For this review, take the finished solid that the model builds, in its own axes (mm). Coordinates: 2 decimals unless noted, no trailing zeros. Order: outer loops, then holes, each group sorted by start corner. A loop starts at its lowest first (then second) coordinate and runs counter-clockwise, first axis right, second up.
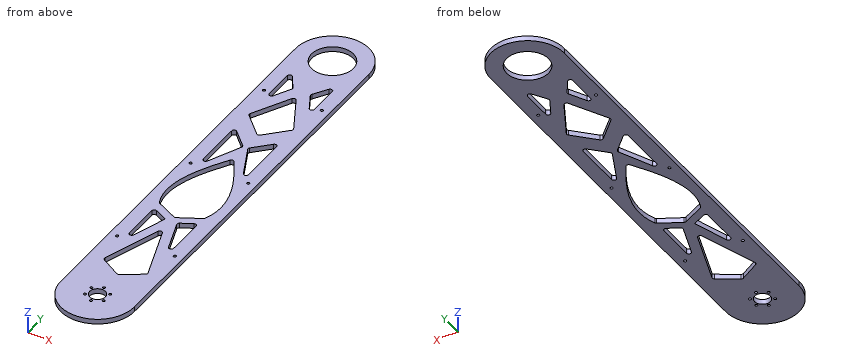
from build123d import *

# Parameters (mm, degrees)
SKETCH2_R           = 10
SKETCH2_R_2         = 1.65
BOSS_EXTRUDE1_DEPTH = 6.35
CUT_EXTRUDE1_DEPTH  = 10
FILLET3_R           = 3
SKETCH5_R           = 1.75
CUT_EXTRUDE2_DEPTH  = 549.511460792
SKETCH6_R           = 26.5
CUT_EXTRUDE3_DEPTH  = 10


with BuildPart() as part:
    # Sketch2 → Boss-Extrude1 (new body)
    with BuildSketch(Plane.XY):
        with BuildLine():
            Line((-46.5, 0), (-46.5, 500))
            ThreePointArc((-46.5, 500), (0, 546.5), (46.5, 500))
            Line((46.5, 500), (46.5, 0))
            ThreePointArc((46.5, 0), (0, -46.5), (-46.5, 0))
        make_face()
        Circle(SKETCH2_R, mode=Mode.SUBTRACT)
        with Locations((0, 13.75)):
            Circle(SKETCH2_R_2, mode=Mode.SUBTRACT)
        with Locations((11.907849302, 6.875)):
            Circle(SKETCH2_R_2, mode=Mode.SUBTRACT)
        with Locations((11.907849302, -6.875)):
            Circle(SKETCH2_R_2, mode=Mode.SUBTRACT)
        with Locations((0, -13.75)):
            Circle(SKETCH2_R_2, mode=Mode.SUBTRACT)
        with Locations((-11.907849302, -6.875)):
            Circle(SKETCH2_R_2, mode=Mode.SUBTRACT)
        with Locations((-11.907849302, 6.875)):
            Circle(SKETCH2_R_2, mode=Mode.SUBTRACT)
    extrude(amount=BOSS_EXTRUDE1_DEPTH)

    # Sketch4 → Cut-Extrude1 (cut)
    with BuildSketch(Plane.XY.offset(6.35)):
        Polygon((28.005258112, 59.37595418), (0, 42.411661153), (-28.005258112, 59.37595418), (0, 141.693437584), align=None)
        Polygon((-7.5, 156.905935087), (-28.005258112, 96.633637735), (-28.005258112, 167.582877854), align=None)
        Polygon((28.005258112, 167.582877854), (7.5, 156.905935087), (28.005258112, 96.633637735), align=None)
        with BuildLine():
            Line((0, 164.275138905), (28.550546746, 179.141206521))
            add(Edge.make_bspline(
                [(28.550546746, 179.141206521), (45.32025339, 216.985654627), (19.430092874, 259.790255689), (0, 290.025756679)],
                knots=[0, 0, 0, 0, 1, 1, 1, 1], degree=3))
            add(Edge.make_bspline(
                [(-28.550546746, 179.141206521), (-45.32025339, 216.985654627), (-19.430092874, 259.790255689), (0, 290.025756679)],
                knots=[0, 0, 0, 0, 1, 1, 1, 1], degree=3))
            Line((-28.550546746, 179.141206521), (0, 164.275138905))
        make_face()
        Polygon((28.550546746, 259.58677623), (3, 314.938284003), (28.550546746, 340.793051053), align=None)
        Polygon((-3, 314.938284003), (-28.550546746, 340.793051053), (-28.550546746, 259.58677623), align=None)
        Polygon((0, 423.142843498), (-28.550546746, 369.246205395), (0, 340.355718526), (28.550546746, 369.246205395), align=None)
        Polygon((-28.550546746, 462.095190817), (-28.550546746, 401.290241252), (-11, 434.421497018), align=None)
        Polygon((28.550546746, 401.290241252), (11, 434.421497018), (28.550546746, 462.095190817), align=None)
    extrude(amount=-CUT_EXTRUDE1_DEPTH, mode=Mode.SUBTRACT)

    # Fillet3
    fillet3_edges = [part.edges().sort_by_distance(p)[0] for p in [
        (-11, 434.421497018, 3.175),
        (-28.550546746, 401.290241252, 3.175),
        (28.550546746, 401.290241252, 3.175),
        (11, 434.421497018, 3.175),
        (28.550546746, 462.095190817, 3.175),
        (-28.550546746, 462.095190817, 3.175),
        (0, 423.142843498, 3.175),
        (-28.550546746, 369.246205395, 3.175),
        (28.550546746, 369.246205395, 3.175),
        (0, 340.355718526, 3.175),
        (28.550546746, 340.793051053, 3.175),
        (-28.550546746, 340.793051053, 3.175),
        (-3, 314.938284003, 3.175),
        (3, 314.938284003, 3.175),
        (28.550546746, 259.58677623, 3.175),
        (-28.550546746, 259.58677623, 3.175),
        (28.550546746, 179.141206521, 3.175),
        (0, 290.025756679, 3.175),
        (-28.550546746, 179.141206521, 3.175),
        (0, 164.275138905, 3.175),
        (-28.005258112, 96.633637735, 3.175),
        (28.005258112, 96.633637735, 3.175),
        (7.5, 156.905935087, 3.175),
        (-28.005258112, 167.582877854, 3.175),
        (28.005258112, 167.582877854, 3.175),
        (0, 141.693437584, 3.175),
        (28.005258112, 59.37595418, 3.175),
        (-28.005258112, 59.37595418, 3.175),
        (0, 42.411661153, 3.175),
    ]]
    fillet(fillet3_edges, radius=FILLET3_R)

    # Sketch5 → Cut-Extrude2 (cut, through all)
    with BuildSketch(Plane.XY.offset(6.35)):
        with Locations((36.5, 103.175)):
            Circle(SKETCH5_R)
        with Locations(Location((-36.5, 103.175, 0), (0, 0, 180))):
            Circle(SKETCH5_R)
        with Locations(Location((36.5, 259.525, 0), (0, 0, 180))):
            Circle(SKETCH5_R)
        with Locations((-36.5, 259.525)):
            Circle(SKETCH5_R)
        with Locations((36.5, 415.875)):
            Circle(SKETCH5_R)
        with Locations(Location((-36.5, 415.875, 0), (0, 0, 180))):
            Circle(SKETCH5_R)
    extrude(amount=-CUT_EXTRUDE2_DEPTH, mode=Mode.SUBTRACT)

    # Sketch6 → Cut-Extrude3 (cut)
    with BuildSketch(Plane.XY.offset(6.35)):
        with Locations((0, 500)):
            Circle(SKETCH6_R)
    extrude(amount=-CUT_EXTRUDE3_DEPTH, mode=Mode.SUBTRACT)


solid = part.part
1. Clearance check with flat-ended pins moving along their axes: pin 1 Ø6 at (x, y) = (23, 269) entering from -Z; pin 2 Ø3 at (x, z) = (-34.5, 5) entering from -Y. State where each tip first meets the part, or that it passes through.
Answer below:
pin 1: stops at z = 0
pin 2: stops at y = -32.76
2. Take a section at A-A, the plane y = 400. Give the boundary of the cut face in (x, z), plus the area to 3 significant figures.
Answer below:
outline: (-46.5, 0) - (-12.26, 0) - (-12.26, 6.35) - (-46.5, 6.35) - close; (12.26, 0) - (46.5, 0) - (46.5, 6.35) - (12.26, 6.35) - close
area: 435 mm2
3. Take a section at B-B, the plane z = 1.25. Give the number of separate pieces and of enclosed holes in the cut face, plus the area to 3 significant figures.
Answer below:
separate pieces: 1
enclosed holes: 23
area: 35,500 mm2
4. To check wall thickness, follow L1, parallel to X at y = 322, z = 4.75; L2, parallel to Y at x = 36.5, z = 2 (3 decimals); L3, parallel to X at y = 448.5, z = 1.75. State the ranges of each line that lie inside material, in increasing order.
Answer below:
L1: x = -46.5 to -28.55, -9.98 to 9.98, 28.55 to 46.5
L2: y = -28.81 to 101.425, 104.925 to 257.775, 261.275 to 414.125, 417.625 to 528.81
L3: x = -46.5 to -28.55, -19.93 to 19.93, 28.55 to 46.5
